Input: part model. Units: mm. Frame: model coordinates. A direction names the side the tool comes from. Give positions to 0.01 mm unless a question says otherwise; leave off trailing zeros. Loops run counter-clockwise (first coordinate to the right, second up) from the corner with the lowest first, then second, coordinate; pieces in that order, holes last. Notation, with made-up numbers: M 75,4 L 87,4 A32 cw 87,34 Z; hole C 47,-20.75 d1. An arc over 180 degrees is marked long. Answer as a JSON object with one key per item and string values. Group by question number.
1) First-contact query: P1, Ø5, axis at x = 4.5, y = -49.5, coming from the +Z side; P2, Ø7, axis at x = 2.5, z = 35, coming from the -Y side; P3, Ø11.5, axis at x = 8.5, y = -28, coming from the -Z side. Flat tips, straight axial feed; report the tip coordinate or a pass-through.
2) Section query A-A on z = -10. Return loops of the section in (x, y), plus the area to 3 significant figures.
3) Access query for faces 1 (the flat face through (12.7, -48, 34)), 2 (the flat face through (-25.4, -50, 1)), 3 (the cylindrical face through (-24.49, -51.51, -24.45)), 4 (the cylindrical face through (-20, -51.51, -24.49)), 5 (the flat face through (0, -65.667, 46)). Directions: +Z, -Z, +X, -X, +Y, -Y. A direction counts if a zero-diameter tool reaches every point of the face in a straight line with its end or side. Return the directions, or none.
4) Section query B-B on x = -4.5. Return loops of the section in (y, z).
5) Section query D-D on x = -11.5. Return loops of the section in (y, z), plus the area to 3 significant figures.
6) Ray query, L1, parallel to X at y = -83.5, z = -4.5; L2, parallel to Z at x = -13, y = -35; L3, parallel to Y at x = -11, z = 30.5. Return the intervals inside material, ascending.
7) Draft query along Z for faces 6 (the flat face through (0, -58.047, 32)), 7 (the cylindrical face through (-0.2, -59.1, 42)), 8 (the flat face through (0, -101.6, 18)), 9 (the cylindrical face through (22.269, -0.554, -24.017)). Return one class per face: +Z half, -Z half, draft (parallel to the pull), parting line (faces both ways), or undercut.
from build123d import *

# Parameters (mm, degrees)
F1_DEPTH      = 101.6
F2_R          = 3.17499
F3_R          = 3.17499
F5_DEPTH      = 12.7
F5_DEPTH_BACK = 12.7
F6_R          = 2.54
F7_R          = 2.54
F8_R          = 2.54
F9_R          = 2.54
F10_R         = 3.81


# Not quite as in the source:
# - a fillet or chamfer is up to 0.001 mm smaller than in the source, because OpenCascade refuses the exact size


with BuildPart() as f1:
    # F0 (on Front) → F1 (new body)
    with BuildSketch(Plane.XZ):
        Polygon((-25.4, 25.4), (-25.4, -25.4), (-19.05, -25.4), (-19.05, 17.78), (19.05, 17.78), (19.05, -25.4), (25.4, -25.4), (25.4, 25.4), align=None)
    extrude(amount=F1_DEPTH)

    # F2 (radius 3.175 in the source; OpenCascade refuses exactly that, so slightly less here)
    f2_edges = [f1.edges().sort_by_distance(p)[0] for p in [
        (-25.4, -50.8, -25.4),
        (-19.05, -50.8, -25.4),
        (-22.225, 0, -25.4),
        (-22.225, -101.6, -25.4),
    ]]
    fillet(f2_edges, radius=F2_R)

    # F3 (radius 3.175 in the source; OpenCascade refuses exactly that, so slightly less here)
    f3_edges = [f1.edges().sort_by_distance(p)[0] for p in [
        (19.05, -50.8, -25.4),
        (25.4, -50.8, -25.4),
        (22.225, 0, -25.4),
        (22.225, -101.6, -25.4),
    ]]
    fillet(f3_edges, radius=F3_R)

    # F4 (on Right) → F5 (join, two sides)
    with BuildSketch(Plane.YZ) as f5_sk:
        Polygon((-58.0474634341, 25.4), (-25.4, 25.4), (-58.0474634341, 48.26), (-65.6674634341, 48.26), (-65.6674634341, 43.18), (-58.0474634341, 43.18), align=None)
    extrude(amount=F5_DEPTH)
    extrude(f5_sk.sketch, amount=-F5_DEPTH_BACK)

    # F6
    f6_edges = [f1.edges().sort_by_distance(p)[0] for p in [
        (25.4, -50.8, 25.4),
    ]]
    fillet(f6_edges, radius=F6_R)

    # F7
    f7_edges = [f1.edges().sort_by_distance(p)[0] for p in [
        (-25.4, -50.8, 25.4),
    ]]
    fillet(f7_edges, radius=F7_R)

    # F8
    f8_edges = [f1.edges().sort_by_distance(p)[0] for p in [
        (-12.7, -41.723732, 36.83),
    ]]
    fillet(f8_edges, radius=F8_R)

    # F9
    f9_edges = [f1.edges().sort_by_distance(p)[0] for p in [
        (12.7, -41.723732, 36.83),
    ]]
    fillet(f9_edges, radius=F9_R)

    # F10
    f10_edges = [f1.edges().sort_by_distance(p)[0] for p in [
        (0, -58.047463, 43.18),
    ]]
    fillet(f10_edges, radius=F10_R)


solid = f1.part
Output:
{
 "1": {"P1": "stops at z = 44.03", "P2": "stops at y = -58.05", "P3": "stops at z = 17.78"},
 "2": {"outline": "M -25.4,-101.6 L -19.05,-101.6 L -19.05,0 L -25.4,0 Z; M 19.05,-101.6 L 25.4,-101.6 L 25.4,0 L 19.05,0 Z", "area": "1,290 mm^2"},
 "3": {"face 1": "+Z, +X, +Y, -Y", "face 2": "+Z, -Z, -X, +Y, -Y", "face 3": "-Z, -X, +Y, -Y", "face 4": "-Z, +Y, -Y", "face 5": "+Z, +X, -X, -Y"},
 "4": {"outline": "M -101.6,17.78 L 0,17.78 L 0,25.4 L -25.4,25.4 L -58.05,48.26 L -65.67,48.26 L -65.67,43.18 L -61.86,43.18 A3.81 cw -58.05,39.37 L -58.05,25.4 L -101.6,25.4 Z"},
 "5": {"outline": "M -101.6,17.78 L 0,17.78 L 0,25.4 L -26.07,25.4 L -58.71,48.26 L -65.67,48.26 L -65.67,43.18 L -61.86,43.18 A3.81 cw -58.05,39.37 L -58.05,25.4 L -101.6,25.4 Z", "area": "1,170 mm^2"},
 "6": {"L1": "x = -25.4 to -19.05, 19.05 to 25.4", "L2": "z = 17.78 to 25.4", "L3": "y = -58.05 to -32.93"},
 "7": {"face 6": "undercut", "face 7": "undercut", "face 8": "draft", "face 9": "-Z half"}
}
